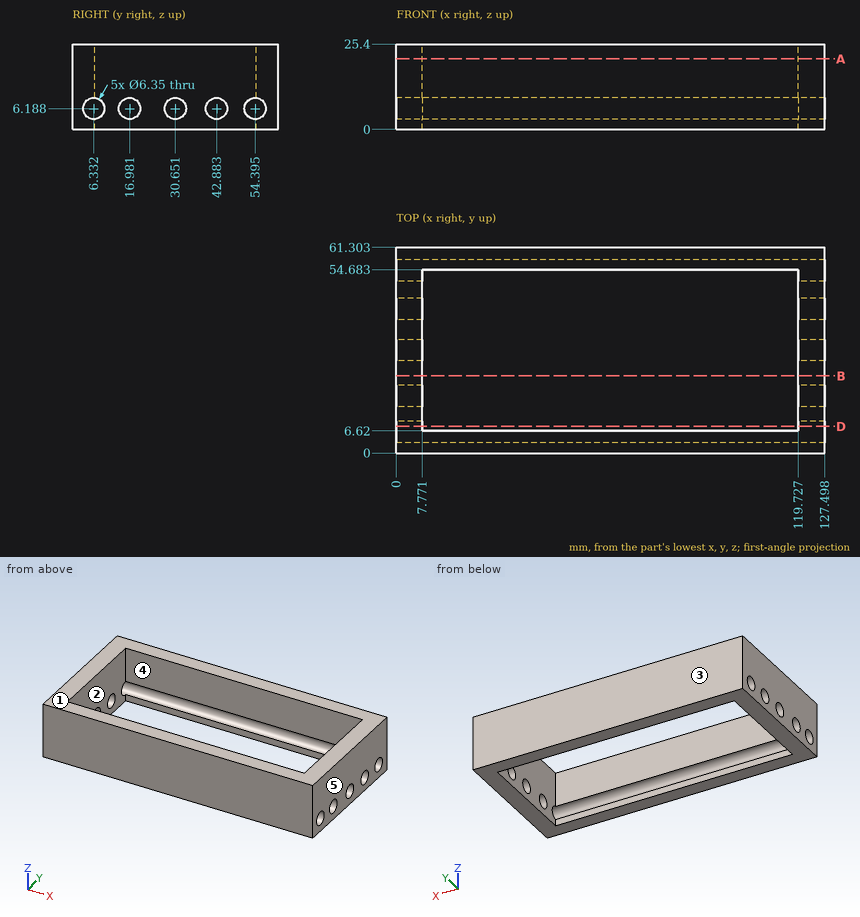
Drawing for the job (mm, zero at the part's lowest x, y, z). A direction names the side the tool comes from. Give positions to 0.01 mm unless a question says otherwise; leave off trailing zeros. Loops run counter-clockwise (first coordinate to the right, second up) from the corner with the lowest first, then second, coordinate; pieces in that order, holes last.
(1) Band-saw the part on B-B (y = 23). Write the cut outline in (x, z).
Return value:
outline: (0, 0) - (7.77, 0) - (7.77, 25.4) - (0, 25.4) - close; (119.73, 0) - (127.5, 0) - (127.5, 25.4) - (119.73, 25.4) - close
(2) Pull direction Y, two halves, no side cores. Call the marked faces 1, 2 and 3: pulls with the +Y half, pulls with the -Y half, needs draft (parallel to the pull), parting line crosses it, or undercut.
Return value:
face 1: needs draft
face 2: undercut
face 3: pulls with the +Y half
(3) 3-axis set-ups, long thin cutter, end or side, ignore diameter. For the marked faces 4 and 5: which of +Z, -Z, +X, -X, +Y, -Y reach the whole face in a straight line?
Return value:
face 4: +Z, -Z
face 5: +Z, -Z, +X, +Y, -Y
(4) Band-saw the part on D-D (y = 8). Write the cut outline in (x, z), and give its area (3 significant figures).
Return value:
outline: (0, 0) - (7.77, 0) - (7.77, 3.49) - (0, 3.49) - close; (0, 8.89) - (7.77, 8.89) - (7.77, 25.4) - (0, 25.4) - close; (119.73, 0) - (127.5, 0) - (127.5, 3.49) - (119.73, 3.49) - close; (119.73, 8.89) - (127.5, 8.89) - (127.5, 25.4) - (119.73, 25.4) - close
area: 311 mm2
(5) Pin check, flat tip, straight feed: pin 1 (5 mm diameter, centred on y = 16.98, z = 6.19, fed in from +X). Stop position of the tip, or through.
Return value:
pin 1: passes through
(6) Band-saw the part on A-A (z = 21). Write the cut outline in (x, y).
Return value:
outline: (0, 0) - (127.5, 0) - (127.5, 61.3) - (0, 61.3) - close; hole (7.77, 6.62) - (119.73, 6.62) - (119.73, 54.68) - (7.77, 54.68) - close
(7) Drill centre lines: line 1 along X through (y, z) = (23, 12.5); line 2 along Y through (x, z) = (104.5, 17.25); line 3 along Y through (x, z) = (120.5, 7.5) (1 decimal). Where is each one in solid material? Low to high.
Return value:
line 1: x = 0 to 7.77, 119.73 to 127.5
line 2: y = 0 to 6.62, 54.68 to 61.3
line 3: y = 0 to 3.4, 9.2 to 14.1, 19.9 to 27.8, 33.5 to 40, 45.8 to 51.5, 57.3 to 61.3
